Input: part model. Units: mm. Frame: model coordinates. Coordinates: 2 decimals unless noted, no trailing zeros. Loops run counter-clockwise (first coordinate to the right, second up) from the corner with the lowest first, then second, coordinate; pieces in that order, holes last. Notation, with made-up numbers: (31, 64.25) - (45, 64.25) arc R21 ccw to (45, 83.25) - close; hole circle Ø4 at (18.25, -17). An arc over 180 degrees is marked (long way). Use one line per item in the form item = value.
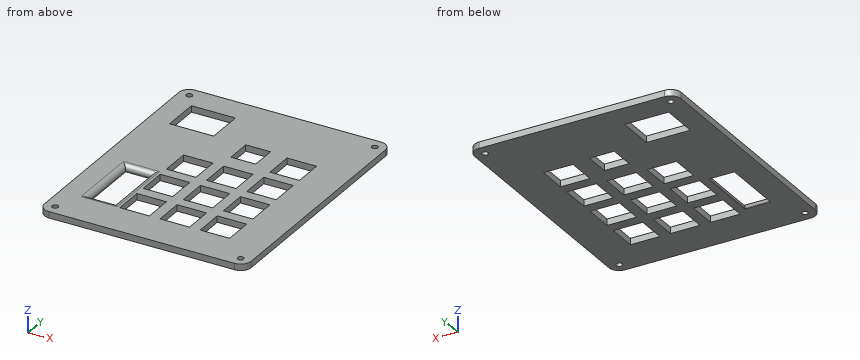
from build123d import *

# Parameters (mm, degrees)
SKETCH6_W           = 119.83
SKETCH6_H           = 98.06
SKETCH6_R           = 1.45
SKETCH6_W_2         = 12.2
SKETCH6_H_2         = 11.8
SKETCH6_W_3         = 13.99955
SKETCH6_H_3         = 13.99955
SKETCH6_W_4         = 29.7
SKETCH6_H_4         = 12.2
SKETCH6_W_5         = 17.85
SKETCH6_H_5         = 20.92
BOSS_EXTRUDE1_DEPTH = 3
FILLET1_R           = 5
FILLET2_R           = 2.5


with BuildPart() as part:
    # Sketch6 → Boss-Extrude1 (new body)
    with BuildSketch(Plane(origin=(0, 0, 0), x_dir=(0, 1, 0), z_dir=(0, 0, 1))):
        with Locations((45.049475, 34.328375)):
            Rectangle(SKETCH6_W, SKETCH6_H)
        with Locations(Location((-9.865525, 78.358375, 0), (0, 0, 270))):
            Circle(SKETCH6_R, mode=Mode.SUBTRACT)
        with Locations(Location((-9.865525, -9.701625, 0), (0, 0, 270))):
            Circle(SKETCH6_R, mode=Mode.SUBTRACT)
        with Locations(Location((99.964475, -9.701625, 0), (0, 0, 270))):
            Circle(SKETCH6_R, mode=Mode.SUBTRACT)
        with Locations(Location((99.964475, 78.358375, 0), (0, 0, 270))):
            Circle(SKETCH6_R, mode=Mode.SUBTRACT)
        with Locations((68.894475, 31.208375)):
            Rectangle(SKETCH6_W_2, SKETCH6_H_2, mode=Mode.SUBTRACT)
        with Locations((28.669475, 28.833375)):
            Rectangle(SKETCH6_W_3, SKETCH6_H_3, mode=Mode.SUBTRACT)
        with Locations((47.719475, 28.833375)):
            Rectangle(SKETCH6_W_3, SKETCH6_H_3, mode=Mode.SUBTRACT)
        with Locations((66.769475, 9.783415)):
            Rectangle(SKETCH6_W_3, SKETCH6_H_3, mode=Mode.SUBTRACT)
        with Locations((47.719475, 9.783415)):
            Rectangle(SKETCH6_W_3, SKETCH6_H_3, mode=Mode.SUBTRACT)
        with Locations((28.669475, 9.783415)):
            Rectangle(SKETCH6_W_3, SKETCH6_H_3, mode=Mode.SUBTRACT)
        with Locations((9.619425, 9.783415)):
            Rectangle(SKETCH6_W_3, SKETCH6_H_3, mode=Mode.SUBTRACT)
        with Locations((9.619425, 28.833375)):
            Rectangle(SKETCH6_W_3, SKETCH6_H_3, mode=Mode.SUBTRACT)
        with Locations((9.619425, 47.883575)):
            Rectangle(SKETCH6_W_3, SKETCH6_H_3, mode=Mode.SUBTRACT)
        with Locations((28.669475, 47.883575)):
            Rectangle(SKETCH6_W_3, SKETCH6_H_3, mode=Mode.SUBTRACT)
        with Locations((47.719475, 47.883575)):
            Rectangle(SKETCH6_W_3, SKETCH6_H_3, mode=Mode.SUBTRACT)
        with Locations((20.17965, 64.843375)):
            Rectangle(SKETCH6_W_4, SKETCH6_H_4, mode=Mode.SUBTRACT)
        with Locations((83.789475, 62.698375)):
            Rectangle(SKETCH6_W_5, SKETCH6_H_5, mode=Mode.SUBTRACT)
    extrude(amount=BOSS_EXTRUDE1_DEPTH)

    # Fillet1
    fillet1_edges = [part.edges().sort_by_distance(p)[0] for p in [
        (-83.358375, 104.964475, 1.5),
        (14.701625, 104.964475, 1.5),
        (14.701625, -14.865525, 1.5),
        (-83.358375, -14.865525, 1.5),
    ]]
    fillet(fillet1_edges, radius=FILLET1_R)

    # Fillet2
    fillet2_edges = [part.edges().sort_by_distance(p)[0] for p in [
        (-64.843375, 5.32965, 3),
        (-58.743375, 20.17965, 3),
        (-64.843375, 35.02965, 3),
        (-70.943375, 20.17965, 3),
    ]]
    fillet(fillet2_edges, radius=FILLET2_R)


solid = part.part
Q1. Ray query, line 1 along Y through (x, z) = (-35, 1.35); line 2 along Y through (x, z) = (-43.5, 1.75); line 3 along X through (y, z) = (52.5, 1.95). Return the intervals inside material, ascending. Write a range as [from, to].
Check values:
line_1 = [-14.87, 2.62], [16.62, 21.67], [35.67, 40.72], [54.72, 62.79], [74.99, 104.96]
line_2 = [-14.87, 2.62], [16.62, 21.67], [35.67, 40.72], [54.72, 104.96]
line_3 = [-83.36, -54.88], [-40.88, -35.83], [-21.83, -16.78], [-2.78, 14.7]
Q2. Cut plane D-D, the plane z = 1.1. Give the number of separate pieces and of enclosed holes in the cut face, then the cut area to 3 significant figures.
Check values:
separate_pieces = 1
enclosed_holes = 17
area = 8,860 mm²
Q3. Cut plane C-C, the plane x = -33.5. Return loops of the section in (y, z).
Check values:
outline = (-14.87, 0) - (2.62, 0) - (2.62, 3) - (-14.87, 3) - close; (16.62, 0) - (21.67, 0) - (21.67, 3) - (16.62, 3) - close; (35.67, 0) - (40.72, 0) - (40.72, 3) - (35.67, 3) - close; (54.72, 0) - (62.79, 0) - (62.79, 3) - (54.72, 3) - close; (74.99, 0) - (104.96, 0) - (104.96, 3) - (74.99, 3) - close
Q4. Cut plane A-A, the plane y = 86.5. Return loops of the section in (x, z), then the cut area to 3 significant figures.
Check values:
outline = (-83.36, 0) - (-73.16, 0) - (-73.16, 3) - (-83.36, 3) - close; (-52.24, 0) - (14.7, 0) - (14.7, 3) - (-52.24, 3) - close
area = 231 mm²
Q5. Cut plane B-B, the plane x = -5.5. Return loops of the section in (y, z), then the cut area to 3 significant figures.
Check values:
outline = (-14.87, 0) - (2.62, 0) - (2.62, 3) - (-14.87, 3) - close; (16.62, 0) - (21.67, 0) - (21.67, 3) - (16.62, 3) - close; (35.67, 0) - (40.72, 0) - (40.72, 3) - (35.67, 3) - close; (54.72, 0) - (59.77, 0) - (59.77, 3) - (54.72, 3) - close; (73.77, 0) - (104.96, 0) - (104.96, 3) - (73.77, 3) - close
area = 191 mm²
